Verification items for the finished model (mm, model axes). A direction names the side the tool comes from. Coordinates: 2 decimals unless noted, no trailing zeros. Write each loop counter-clockwise with the first axis right and the second up, starting at its lowest first coordinate (ties: lowest second). Pieces come first, ordered by that corner, then holes. Notation, with made-up numbers: M -12.5,-9.75 L 13.5,-9.75 A24 ccw 13.5,27.25 Z; hole C -4,72.25 d2. An arc over 180 degrees is marked long. One line per item, written item: value.
```python
from build123d import *

# Parameters (mm, degrees)
SKETCH1_R           = 5
BOSS_EXTRUDE1_DEPTH = 7
SKETCH1_3_R         = 0.75
SKETCH1_3_R_2       = 0.37500000000000105
SKETCH1_3_R_3       = 0.375000000000001
SKETCH1_3_R_4       = 0.7500000000000001
BOSS_EXTRUDE2_DEPTH = 3.2
CHAMFER1_SIZE       = 0.5


with BuildPart() as part:
    # Sketch1 → Boss-Extrude1 (new body)
    with BuildSketch(Plane.XY):
        with BuildLine():
            ThreePointArc((-7.67241426287147, 9.226811983501475), (-9.846222893058407, 6.8594383691533025), (-11.31370849898476, 4))
            ThreePointArc((-11.31370849898476, 4), (-12, 1.47e-15), (-11.313708498984761, -3.9999999999999973))
            ThreePointArc((-11.313708498984761, -3.9999999999999973), (-9.846222893058428, -6.859438369153274), (-7.672414262871522, -9.226811983501433))
            ThreePointArc((-7.672414262871518, -9.226811983501431), (-7.566872377799013, -9.309109229750973), (-7.464748895834485, -9.395611950380768))
            ThreePointArc((-7.464748895834483, -9.395611950380767), (1.911e-14, -12), (7.464748895834521, -9.395611950380736))
            ThreePointArc((7.464748895834522, -9.395611950380738), (7.566872377798977, -9.309109229751012), (7.6724142628714045, -9.226811983501536))
            ThreePointArc((7.672414262871396, -9.226811983501538), (10.864367702596793, -5.0956368024783405), (12, -2.94e-15))
            ThreePointArc((12, 0), (10.864367702596812, 5.095636802478297), (7.672414262871458, 9.226811983501484))
            ThreePointArc((7.672414262871453, 9.22681198350148), (7.5668723777987985, 9.309109229751144), (7.4647488958341315, 9.395611950381072))
            ThreePointArc((7.464748895834118, 9.395611950381056), (-2.7638e-13, 12), (-7.464748895834552, 9.395611950380712))
            ThreePointArc((-7.464748895834552, 9.395611950380712), (-7.566872377799023, 9.30910922975097), (-7.672414262871468, 9.226811983501477))
        make_face()
        Circle(SKETCH1_R, mode=Mode.SUBTRACT)
    extrude(amount=BOSS_EXTRUDE1_DEPTH)

    # Sketch1<3> → Boss-Extrude2 (add)
    # profile 1 of 3: a face of its own
    with BuildSketch(Plane.XY):
        with BuildLine():
            ThreePointArc((-6.57839458957231, 13.089966563130929), (-6.4376977661817865, 11.10270546197924), (-7.464748895834552, 9.395611950380712))
            ThreePointArc((-7.464748895834552, 9.395611950380712), (-2.7638e-13, 12), (7.464748895834118, 9.395611950381056))
            ThreePointArc((7.4647488958341315, 9.395611950381072), (6.437697766181707, 11.102705461979504), (6.578394589572291, 13.089966563130933))
            ThreePointArc((6.578394589572291, 13.089966563130933), (6.498593335336791, 15.184618723292306), (4.899264696142665, 16.53964042647633))
            ThreePointArc((4.899264696142668, 16.539640426476332), (-9.55e-15, 17.250000000000007), (-4.899264696142684, 16.539640426476325))
            ThreePointArc((-4.899264696142685, 16.539640426476325), (-6.49859333533681, 15.184618723292303), (-6.57839458957231, 13.089966563130929))
        make_face()
        with Locations((-4.160824799912482, 14.046709115819024)):
            Circle(SKETCH1_3_R, mode=Mode.SUBTRACT)
        with BuildLine():
            ThreePointArc((-2e-17, 13.55), (-1.1000000000000003, 14.65), (1.8e-16, 15.75))
            ThreePointArc((1.8e-16, 15.75), (2.734958798254155, 15.510722109942275), (5.3868172573792865, 14.800158777378059))
            ThreePointArc((5.3868172573792865, 14.800158777378059), (6.04425698258554, 13.390274736855329), (4.634372942062814, 12.732835011649062))
            ThreePointArc((4.634372942062814, 12.732835011649065), (2.352932807386907, 13.344145053315419), (-2e-17, 13.550000000000002))
        make_face(mode=Mode.SUBTRACT)
    # profile 2 of 3: a face of its own
    with BuildSketch(Plane.XY):
        with BuildLine():
            Line((-11.313708498984761, 3.9999999999999982), (-16.2, 4))
            Line((-16.2, 4), (-16.2, -4))
            Line((-16.2, -4), (-11.313708498984761, -3.9999999999999982))
            ThreePointArc((-11.313708498984761, -3.9999999999999973), (-12, 1.47e-15), (-11.31370849898476, 4))
        make_face()
        with Locations((-14.7, -2.5)):
            Circle(SKETCH1_3_R_2, mode=Mode.SUBTRACT)
        with Locations((-14.7, 0)):
            Circle(SKETCH1_3_R_3, mode=Mode.SUBTRACT)
        with Locations((-14.7, 2.5)):
            Circle(SKETCH1_3_R_2, mode=Mode.SUBTRACT)
    # profile 3 of 3: a face of its own
    with BuildSketch(Plane.XY):
        with BuildLine():
            ThreePointArc((7.464748895834521, -9.395611950380736), (1.911e-14, -12), (-7.464748895834483, -9.395611950380767))
            ThreePointArc((-7.464748895834485, -9.395611950380768), (-6.437697766181827, -11.102705461979276), (-6.578394589572382, -13.08996656313089))
            ThreePointArc((-6.578394589572383, -13.08996656313089), (-6.498593335336874, -15.184618723292306), (-4.899264696142685, -16.539640426476325))
            ThreePointArc((-4.899264696142686, -16.539640426476325), (-2e-15, -17.250000000000004), (4.899264696142684, -16.53964042647633))
            ThreePointArc((4.899264696142683, -16.539640426476325), (6.498593335336733, -15.184618723292296), (6.57839458957222, -13.089966563130977))
            ThreePointArc((6.57839458957222, -13.089966563130977), (6.437697766181717, -11.102705461979264), (7.464748895834522, -9.395611950380738))
        make_face()
        with BuildLine():
            ThreePointArc((-4.634372942062905, -12.732835011649033), (-2.3529328073870017, -13.344145053315408), (-9.46e-14, -13.550000000000006))
            ThreePointArc((-9.46e-14, -13.550000000000004), (1.099999999999898, -14.650000000000011), (-1.1017e-13, -15.750000000000004))
            ThreePointArc((-1.1017e-13, -15.750000000000004), (-2.734958798254263, -15.510722109942261), (-5.3868172573793895, -14.800158777378023))
            ThreePointArc((-5.3868172573793895, -14.800158777378021), (-6.044256982585632, -13.390274736855288), (-4.634372942062904, -12.73283501164903))
        make_face(mode=Mode.SUBTRACT)
        with Locations((4.160824799912384, -14.046709115819057)):
            Circle(SKETCH1_3_R_4, mode=Mode.SUBTRACT)
    extrude(amount=BOSS_EXTRUDE2_DEPTH)

    # Chamfer1
    # the kernel refuses this chamfer: 0.5 mm, written as the material it takes off along each edge
    with BuildSketch(Plane(origin=(4.4e-16, 8.88e-15, 7), x_dir=(-0.7022542311891906, -0.7119262565581345, 0), z_dir=(-0.7119262565581345, 0.7022542311891906, 0))) as chamfer1_piece_1:
        Polygon((12.00000000000001, -CHAMFER1_SIZE), (12.00000000000001 - CHAMFER1_SIZE, 0), (12.00000000000001, 0), align=None)
    revolve(axis=Axis((4.4e-16, 8.88e-15, 7), (0, 0, 1)), revolution_arc=89.21628448783436, mode=Mode.SUBTRACT)
    with BuildSketch(Plane(origin=(0, -1.55e-15, 7), x_dir=(0.5534232565861029, 0.8329001735319981, 0), z_dir=(-0.8329001735319981, 0.5534232565861029, 0))) as chamfer1_piece_2:
        Polygon((12.000000000000009, CHAMFER1_SIZE), (12.000000000000009 - CHAMFER1_SIZE, 0), (12.000000000000009, 0), align=None)
    revolve(axis=Axis((0, -1.55e-15, 7), (0, 0, -1)), revolution_arc=112.79563771505457, mode=Mode.SUBTRACT)
    with BuildSketch(Plane(origin=(0, 0, 7), x_dir=(0.7022542311891632, 0.7119262565581616, 0), z_dir=(0.7119262565581616, -0.7022542311891632, 0))) as chamfer1_piece_3:
        Polygon((12.000000000000002, -CHAMFER1_SIZE), (12.000000000000002 - CHAMFER1_SIZE, 0), (12.000000000000002, 0), align=None)
    revolve(axis=Axis((0, 0, 7), (0, 0, 1)), revolution_arc=89.2162844878324, mode=Mode.SUBTRACT)
    with BuildSketch(Plane(origin=(-2.309e-14, -1.688e-14, 7), x_dir=(-0.5534232565861079, -0.8329001735319947, 0), z_dir=(0.8329001735319947, -0.5534232565861079, 0))) as chamfer1_piece_4:
        Polygon((12.00000000000003, CHAMFER1_SIZE), (12.00000000000003 - CHAMFER1_SIZE, 0), (12.00000000000003, 0), align=None)
    revolve(axis=Axis((-2.309e-14, -1.688e-14, 7), (0, 0, -1)), revolution_arc=112.79563771505396, mode=Mode.SUBTRACT)


solid = part.part
```
Item 1: Go/stop test with flat-tipped pins: P1, Ø3.5, axis at x = -13.5, z = 1, coming from the -Y side; P2, Ø1, axis at y = 12, z = 1.5, coming from the -X side; P3, Ø4, axis at y = 9, z = 2, coming from the +X side. Record where each tip stops, or that it passes through.
The answers:
P1: stops at y = -4
P2: stops at x = -6.41
P3: stops at x = 9.75
Item 2: Cross-section at A-A, the plane x = -14.7. Enter the section's corners in (y, z) (3 decimals), and give its area (3 significant figures).
The answers:
outline: M -4,0 L -2.875,0 L -2.875,3.2 L -4,3.2 Z; M -2.125,0 L -0.375,0 L -0.375,3.2 L -2.125,3.2 Z; M 0.375,0 L 2.125,0 L 2.125,3.2 L 0.375,3.2 Z; M 2.875,0 L 4,0 L 4,3.2 L 2.875,3.2 Z
area: 18.4 mm²
Item 3: Draft check along Y on faces 1 (the face through (12, 0, 3)), 2 (the face through (-2.697, -15.517, 1.578)), 3 (the face through (2, -5, 7)). Enter one of: released by +Y, released by -Y, zero draft, split by the parting line, or undercut.
The answers:
face 1: split by the parting line
face 2: undercut
face 3: zero draft
Item 4: Access from +Z, -Z, +X, -X, +Y, -Y to the whole of each face (thin tool, end or side, straight path). Record for faces 4 (the face through (-6.648, -10.495, 1.761)), 5 (the face through (2.697, 15.517, 1.578)).
The answers:
face 4: +Z, -Z, -X
face 5: +Z, -Z
Item 5: Cross-section at D-D, the plane z = 2.5. Give the number of separate pieces and of enclosed holes in the cut face, and give its area (3 significant figures).
The answers:
separate pieces: 1
enclosed holes: 8
area: 516 mm²
Item 6: Scan lines: line 1 (Y direction, x = -14.7, z = 0.9) (3 decimals); line 2 (Y direction, x = 0, z = 3); line 3 (Y direction, x = -2, z = 0.5). Record each from-to range of solid material in increasing order.
The answers:
line 1: y = -4 to -2.875, -2.125 to -0.375, 0.375 to 2.125, 2.875 to 4
line 2: y = -17.25 to -15.75, -13.55 to -5, 5 to 13.55, 15.75 to 17.25
line 3: y = -17.13 to -15.62, -13.4 to -4.58, 4.58 to 17.13
Item 7: Cross-section at C-C, the plane z = 4.75. Enter the section's corners in (x, y).
The answers:
outline: M -7.67,-9.23 A3.31 cw -7.46,-9.4 A12 ccw 7.46,-9.4 A3.31 cw 7.67,-9.23 A12 ccw 7.67,9.23 A3.31 cw 7.46,9.4 A12 ccw -7.46,9.4 A3.31 cw -7.67,9.23 A12 ccw Z; hole C 0,0 d10
Item 8: Cross-section at B-B, the plane y = 0. Enter the section's corners in (x, z) (3 decimals), and give its area (3 significant figures).
The answers:
outline: M -16.2,0 L -15.075,0 L -15.075,3.2 L -16.2,3.2 Z; M -14.325,0 L -5,0 L -5,7 L -11.5,7 L -12,6.5 L -12,3.2 L -14.325,3.2 Z; M 5,0 L 12,0 L 12,6.5 L 11.5,7 L 5,7 Z
area: 109 mm²
